For this review, take the finished solid that the model builds, in its own axes (mm). A direction names the side the tool comes from. Round coordinates to 2 decimals unless told otherwise and drop trailing zeros. Order: outer loops, then holes, each group sorted by start corner. A loop starts at its lowest first (then second) coordinate and runs counter-clockwise, first axis right, second up. Notation, with made-up numbers: (88, -37) - (116, -37) arc R19 cw to (116, -22) - close; hole circle Ø4 at (-17, 51). An arc over 180 degrees is marked (long way). One line per item, written item: value.
```python
from build123d import *

# Parameters (mm, degrees)
SKETCH2_W                        = 60
SKETCH2_H                        = 60
BOSS_EXTRUDE1_DEPTH              = 10
SKETCH7_W                        = 28.32
SKETCH7_H                        = 16.5
CUT_EXTRUDE2_DEPTH               = 44.588989435
FILLET2_R                        = 2
CBORE_FOR_M2_5_SHCS2_D           = 3.1
CBORE_FOR_M2_5_SHCS2_CBORE_D     = 5.5
CBORE_FOR_M2_5_SHCS2_CBORE_DEPTH = 2.5
MOVE_FACE1_BY                    = 3.5
MOVE_FACE1_2_BY                  = 3.5
MOVE_FACE1_3_BY                  = 3.5
MOVE_FACE1_4_BY                  = 3.5
SKETCH11_W                       = 10
SKETCH11_H                       = 44.7
BOSS_EXTRUDE2_DEPTH              = 60
SKETCH12_W                       = 20
SKETCH12_H                       = 60
BOSS_EXTRUDE3_DEPTH              = 10
CBORE_FOR_M4_SHCS1_D             = 4.8
CBORE_FOR_M4_SHCS1_CBORE_D       = 8
CBORE_FOR_M4_SHCS1_CBORE_DEPTH   = 4
FILLET5_R                        = 2


with BuildPart() as part:
    # Sketch2 → Boss-Extrude1 (new body)
    with BuildSketch(Plane(origin=(0, 0, 0), x_dir=(1, 0, 0), z_dir=(0, 1, 0))):
        Rectangle(SKETCH2_W, SKETCH2_H)
    extrude(amount=BOSS_EXTRUDE1_DEPTH)

    # Sketch7 → Cut-Extrude2 (cut, through all)
    with BuildSketch(Plane(origin=(0, 10, 0), x_dir=(1, 0, 0), z_dir=(0, 1, 0))):
        Rectangle(SKETCH7_W, SKETCH7_H)
    extrude(amount=-CUT_EXTRUDE2_DEPTH, mode=Mode.SUBTRACT)

    # Fillet2
    fillet2_edges = [part.edges().sort_by_distance(p)[0] for p in [
        (-14.16, 5, 8.25),
        (-14.16, 5, -8.25),
        (14.16, 5, -8.25),
        (14.16, 5, 8.25),
    ]]
    fillet(fillet2_edges, radius=FILLET2_R)

    # CBORE for M2.5 SHCS2 (through all)
    with Locations(Plane(origin=(0, 0, 0), x_dir=(-1, 0, 0), z_dir=(0, -1, 0))):
        with Locations((11, -20), (-11, -20), (11, 20), (-11, 20)):
            CounterBoreHole(CBORE_FOR_M2_5_SHCS2_D / 2, CBORE_FOR_M2_5_SHCS2_CBORE_D / 2, CBORE_FOR_M2_5_SHCS2_CBORE_DEPTH)

    # Move Face1: a face moved inward by 3.5
    extrude(part.faces().sort_by_distance((11, 2.5, -17.8))[0], amount=MOVE_FACE1_BY, dir=(0, 1, 0), mode=Mode.SUBTRACT)

    # Move Face1 2: a face moved inward by 3.5
    extrude(part.faces().sort_by_distance((-11, 2.5, -17.8))[0], amount=MOVE_FACE1_2_BY, dir=(0, 1, 0), mode=Mode.SUBTRACT)

    # Move Face1 3: a face moved inward by 3.5
    extrude(part.faces().sort_by_distance((11, 2.5, 22.2))[0], amount=MOVE_FACE1_3_BY, dir=(0, 1, 0), mode=Mode.SUBTRACT)

    # Move Face1 4: a face moved inward by 3.5
    extrude(part.faces().sort_by_distance((-11, 2.5, 22.2))[0], amount=MOVE_FACE1_4_BY, dir=(0, 1, 0), mode=Mode.SUBTRACT)

    # Sketch11 → Boss-Extrude2 (add)
    with BuildSketch(Plane(origin=(0, 0, -30), x_dir=(-1, 0, 0), z_dir=(0, 0, -1))):
        with Locations((-25, -22.35)):
            Rectangle(SKETCH11_W, SKETCH11_H)
    boss_extrude2 = extrude(amount=-BOSS_EXTRUDE2_DEPTH)

    # Sketch12 → Boss-Extrude3 (add)
    with BuildSketch(Plane.XZ.offset(44.7)):
        with Locations((40, 0)):
            Rectangle(SKETCH12_W, SKETCH12_H)
    boss_extrude3 = extrude(amount=-BOSS_EXTRUDE3_DEPTH)

    # CBORE for M4 SHCS1 (through all)
    with Locations(Plane(origin=(0, -34.7, 0), x_dir=(1, 0, 0), z_dir=(0, 1, 0))):
        with Locations((40, 20), (40, -20)):
            cbore_for_m4_shcs1 = CounterBoreHole(CBORE_FOR_M4_SHCS1_D / 2, CBORE_FOR_M4_SHCS1_CBORE_D / 2, CBORE_FOR_M4_SHCS1_CBORE_DEPTH)

    # Mirror1: Boss-Extrude2, Boss-Extrude3, CBORE for M4 SHCS1 across plane
    add(boss_extrude2.mirror(Plane(origin=(0, 0, 0), x_dir=(0, 0, 1), z_dir=(1, 0, 0))))
    add(boss_extrude3.mirror(Plane(origin=(0, 0, 0), x_dir=(0, 0, 1), z_dir=(1, 0, 0))))
    add(cbore_for_m4_shcs1.mirror(Plane(origin=(0, 0, 0), x_dir=(0, 0, 1), z_dir=(1, 0, 0))), mode=Mode.SUBTRACT)

    # Fillet5
    fillet5_edges = [part.edges().sort_by_distance(p)[0] for p in [
        (50, -34.7, 0),
        (30, -34.7, 0),
        (30, 10, 0),
        (-20, 0, 0),
        (-20, -44.7, 0),
        (-30, -34.7, 0),
        (-50, -34.7, 0),
        (-30, 10, 0),
        (20, 0, 0),
        (20, -44.7, 0),
    ]]
    fillet(fillet5_edges, radius=FILLET5_R)


solid = part.part
```
Item 1: Take a section at A-A (y = -22). Write out the cut boundary in (x, z), plus the area to 3 significant figures.
Returned:
outline: (-30, -30) - (-20, -30) - (-20, 30) - (-30, 30) - close; (20, -30) - (30, -30) - (30, 30) - (20, 30) - close
area: 1,200 mm^2
Item 2: Machinability: for faces 4 (the cylindrical face through (37.05, -36.67, 17.3)), 5 (the flat face through (0, 5, 8.25)), 6 (the cylindrical face through (-19.43, -0.6, 0.42)), 7 (the flat face through (-40, -34.7, 0)), 8 (the flat face through (40, -34.7, 0)), which of the approach directions +Z, -Z, +X, -X, +Y, -Y give a long, thin tool a straight path to every point of the face, cutting with its end or side? Answer none if there is none.
Returned:
face 4: +Y
face 5: +Y, -Y
face 6: +Z, -Z, -Y
face 7: +Z, -Z, -X, +Y
face 8: +Z, -Z, +X, +Y
Item 3: Take a section at B-B (z = -2.5). Write out the cut boundary in (x, y).
Returned:
outline: (-50, -44.7) - (-22, -44.7) arc R2 ccw to (-20, -42.7) - (-20, -2) arc R2 cw to (-18, 0) - (-14.16, 0) - (-14.16, 10) - (-28, 10) arc R2 ccw to (-30, 8) - (-30, -32.7) arc R2 cw to (-32, -34.7) - (-48, -34.7) arc R2 ccw to (-50, -36.7) - close; (14.16, 0) - (18, 0) arc R2 cw to (20, -2) - (20, -42.7) arc R2 ccw to (22, -44.7) - (50, -44.7) - (50, -36.7) arc R2 ccw to (48, -34.7) - (32, -34.7) arc R2 cw to (30, -32.7) - (30, 8) arc R2 ccw to (28, 10) - (14.16, 10) - close
Item 4: Take a section at D-D (x = -11). Write out the cut boundary in (y, z).
Returned:
outline: (0, -30) - (10, -30) - (10, -21.55) - (6, -21.55) - (6, -22.75) - (0, -22.75) - close; (0, -17.25) - (6, -17.25) - (6, -18.45) - (10, -18.45) - (10, -8.25) - (0, -8.25) - close; (0, 8.25) - (10, 8.25) - (10, 18.45) - (6, 18.45) - (6, 17.25) - (0, 17.25) - close; (0, 22.75) - (6, 22.75) - (6, 21.55) - (10, 21.55) - (10, 30) - (0, 30) - close
Item 5: The part is to be moulded in two halves that separate along Z. For faces 1 (the flat face through (-20, -23, 0)), 2 (the cylindrical face through (-11.202, 8.028, 18.463)), 3 (the flat face through (1, 1, -30)), say which applies: +Z half, -Z half, draft (parallel to the pull), parting line (faces both ways), or undercut.
Returned:
face 1: draft
face 2: undercut
face 3: -Z half
Item 6: For P1, Ø1, axis at x = 19, z = 8, coming from the -Y side; P2, Ø3, axis at y = -18.5, z = -15.5, coming from the -X side; P3, Ø10.5, axis at x = 40, z = 20, coming from the +Y side; P4, Ø4.5, axis at x = -40, z = -20, coming from the -Y side, all flat-tipped, find the tip position at first contact; note any pin that passes through.
Returned:
P1: y = -0.68
P2: x = -30
P3: y = -34.7
P4: through
Item 7: Wall thickness on line 1 (X direction, y = 4, z = 20); line 2 (X direction, y = -37.35, z = -20); line 3 (Z direction, x = -40, y = -43): over which ranges is each line inside the solid? List them lowest first.
Returned:
line 1: -30 to -13.75, -8.25 to 8.25, 13.75 to 30
line 2: -50 to -44, -36 to -20, 20 to 36, 44 to 50
line 3: -30 to -22.4, -17.6 to 17.6, 22.4 to 30
Item 8: Take a section at C-C (x = 40). Write out the cut boundary in (y, z).
Returned:
outline: (-44.7, -30) - (-34.7, -30) - (-34.7, -24) - (-38.7, -24) - (-38.7, -22.4) - (-44.7, -22.4) - close; (-44.7, -17.6) - (-38.7, -17.6) - (-38.7, -16) - (-34.7, -16) - (-34.7, 16) - (-38.7, 16) - (-38.7, 17.6) - (-44.7, 17.6) - close; (-44.7, 22.4) - (-38.7, 22.4) - (-38.7, 24) - (-34.7, 24) - (-34.7, 30) - (-44.7, 30) - close
